Model file for the job. Use its own axes, mm. A direction names the side the tool comes from. Give positions to 0.01 mm unless a question says otherwise; leave off trailing zeros. Loops run counter-clockwise (first coordinate to the right, second up) from the corner with the lowest first, then second, coordinate; pieces in that order, holes last. Notation, with made-up numbers: (33, 74.25) - (67, 74.25) arc R12 cw to (67, 97.25) - close; hole circle Ø1 at (66, 64.5). An arc over 180 degrees is marked (long way). Use a Markdown table: item, result.
from build123d import *

# Parameters (mm, degrees)
BOSS_EXTRUDE1_DEPTH = 9.525
BOSS_EXTRUDE2_DEPTH = 4.7625


with BuildPart() as part:
    # Sketch1 → Boss-Extrude1 (new body)
    with BuildSketch(Plane(origin=(0, 0, 0), x_dir=(1, 0, 0), z_dir=(0, 1, 0))):
        with BuildLine():
            Line((0, 0), (0, -19.05))
            ThreePointArc((0, -19.05), (91.91625, -32.645980635), (183.8325, -19.05))
            Line((183.8325, -19.05), (183.8325, 0))
            Line((183.8325, 0), (145.7325, 0))
            ThreePointArc((145.7325, 0), (91.91625, -22.253255558), (38.1, 0))
            Line((38.1, 0), (0, 0))
        make_face()
    extrude(amount=BOSS_EXTRUDE1_DEPTH)

    # Sketch2 → Boss-Extrude2 (add, symmetric)
    with BuildSketch(Plane(origin=(91.91625, 0, 0), x_dir=(0, 0, -1), z_dir=(1, 0, 0))):
        Polygon((-32.645980635, 0), (-32.645980635, -6.35), (-27.581538216, -6.35), (-22.253255558, 0), align=None)
    extrude(amount=BOSS_EXTRUDE2_DEPTH, both=True)


solid = part.part
(1) Drill centre lines: probe 1 along Y at (x, z) = (36, 10) (3 decimals); probe 2 along X at (y, z) = (3.75, 2); probe 3 along X at (y, z) = (5, 16). Where is each one in solid material? Low to high. Write a range as [from, to].
Computed:
| item | result |
|---|---|
| probe 1 | [0, 9.525] |
| probe 2 | [0, 40.18], [143.65, 183.83] |
| probe 3 | [0, 61.69], [122.15, 183.83] |
(2) Pin check, flat tips, straight feed: P1, Ø3, axis at y = -2, z = 26.5, coming from the +X side; P2, Ø7, axis at y = -4, z = 28, coming from the -X side; P3, Ø16.5, axis at x = 59, z = 12.5, coming from the -Y side; P4, Ø4, axis at x = 158, z = 28, coming from the -Y side. Stop position of each tip, or through.
Computed:
| item | result |
|---|---|
| P1 | x = 96.68 |
| P2 | x = 87.15 |
| P3 | y = 0 |
| P4 | through |
(3) Slice it at C-C, the plane z = 14. Write the cut outline in (x, y) (1 decimal), plus the area to 3 significant figures.
Computed:
| item | result |
|---|---|
| outline | (0, 0) - (57.4, 0) - (57.4, 9.5) - (0, 9.5) - close; (126.4, 0) - (183.8, 0) - (183.8, 9.5) - (126.4, 9.5) - close |
| area | 1,090 mm² |
(4) 3-axis set-ups, long thin cutter, end or side, ignore diameter. For faces 4 (the flat face through (147, 0, 16)), 5 (the flat face through (91.983, -3.219, 24.955)), 6 (the flat face through (35, 0, 16)): which of +Z, -Z, +X, -X, +Y, -Y reach the whole face in a straight line?
Computed:
| item | result |
|---|---|
| face 4 | +Z, -Z, +X, -Y |
| face 5 | -Z, +X, -X, -Y |
| face 6 | +Z, -Z, -X, -Y |
(5) Mould opens along X. For faces 1 (the flat face through (96.679, -3, 29)), 2 (the cylindrical face through (92.75, 4.7, 22.25)), 3 (the flat face through (19, 5, 0)) say: pulls with the +X half, pulls with the -X half, needs draft (parallel to the pull), parting line crosses it, or undercut.
Computed:
| item | result |
|---|---|
| face 1 | pulls with the +X half |
| face 2 | undercut |
| face 3 | needs draft |
(6) Slice it at A-A, the plane z = 6. Write the cut outline in (x, y) (1 decimal), plus the area to 3 significant figures.
Computed:
| item | result |
|---|---|
| outline | (0, 0) - (44.9, 0) - (44.9, 9.5) - (0, 9.5) - close; (139, 0) - (183.8, 0) - (183.8, 9.5) - (139, 9.5) - close |
| area | 855 mm² |
(7) Slice it at B-B, the plane y = 3.25. Write the cut outline in (x, z), plus the area to 3 significant figures.
Computed:
| item | result |
|---|---|
| outline | (0, 0) - (38.1, 0) arc R76.2 cw to (145.73, 0) - (183.83, 0) - (183.83, 19.05) arc R317.5 ccw to (0, 19.05) - close |
| area | 3,530 mm² |
(8) Slice it at D-D, the plane x = 12. Write the cut outline in (y, z) (3 decimals), plus the area to 3 significant figures.
Computed:
| item | result |
|---|---|
| outline | (0, 0) - (9.525, 0) - (9.525, 22.424) - (0, 22.424) - close |
| area | 214 mm² |
